Input: part model. Units: mm. Frame: model coordinates. Face numbers are marked on the shaded views. A direction names the side the tool comes from. Round coordinates to 2 decimals unless told otherwise and drop trailing zeros. Order: outer loops, then holes, each group sorted by start corner. A loop starts at its lowest first (then second) coordinate and runs counter-clockwise, first axis right, second up. Notation, with made-up numbers: (-38.5, 31.25) -> (-4.5, 31.25) arc R12 ccw to (-4.5, 41.25) -> close; hole circle Ø11 at (-5, -40). An arc over 180 degrees is marked (long way). Use a Markdown table: item, result.
from build123d import *

# Parameters (mm, degrees)
BOSS_EXTRUDE1_DEPTH = 6
FILLET1_R           = 20
SKETCH4_W           = 3
SKETCH4_H           = 8
SKETCH6_R           = 16.245672788
CUT_EXTRUDE1_DEPTH  = 10


with BuildPart() as part:
    # Sketch1 → Boss-Extrude1 (new body)
    with BuildSketch(Plane(origin=(0, 0, 0), x_dir=(1, 0, 0), z_dir=(0, 1, 0))):
        with BuildLine():
            Line((34.540516942, 38.609131748), (-36.459483058, 38.609131748))
            ThreePointArc((-36.459483058, 38.609131748), (-66.459483058, 1.109131748), (-36.459483058, -36.390868252))
            Line((-36.459483058, -36.390868252), (34.540516942, -36.390868252))
            ThreePointArc((34.540516942, -36.390868252), (64.540516942, 1.109131748), (34.540516942, 38.609131748))
        make_face()
    extrude(amount=BOSS_EXTRUDE1_DEPTH)

    # Fillet1
    fillet1_edges = [part.edges().sort_by_distance(p)[0] for p in [
        (-36.459483058, 3, -38.609131748),
        (34.540516942, 3, -38.609131748),
        (34.540516942, 3, 36.390868252),
        (-36.459483058, 3, 36.390868252),
    ]]
    fillet(fillet1_edges, radius=FILLET1_R)

    # Sweep1: sweep along a path in Sketch3
    with BuildLine(Plane.XZ) as sweep1_path:
        Line((31.907446823, 29.390868252), (-33.82641294, 29.390868252))
        ThreePointArc((-33.82641294, 29.390868252), (-35.899239553, 29.224550102), (-37.919027907, 28.729851303))
        ThreePointArc((-37.919027907, 28.729851303), (-59.459483058, -1.109131748), (-37.919027907, -30.948114799))
        ThreePointArc((-37.919027907, -30.948114799), (-35.899239553, -31.442813598), (-33.82641294, -31.609131748))
        Line((-33.82641294, -31.609131748), (31.907446823, -31.609131748))
        ThreePointArc((31.907446823, -31.609131748), (33.980273437, -31.442813598), (36.000061791, -30.948114799))
        ThreePointArc((36.000061791, -30.948114799), (57.540516942, -1.109131748), (36.000061791, 28.729851303))
        ThreePointArc((36.000061791, 28.729851303), (33.980273437, 29.224550102), (31.907446823, 29.390868252))
    # Sketch4 → Sweep1 (sweep)
    with BuildSketch(Plane(origin=(31.907446823, 0, -31.609131748), x_dir=(0, 0, -1), z_dir=(1, 0, 0))):
        with Locations((-1.5, -4)):
            Rectangle(SKETCH4_W, SKETCH4_H)
    sweep(path=sweep1_path.line)

    # Sketch6 → Cut-Extrude1 (cut)
    with BuildSketch(Plane(origin=(0, 0, 0), x_dir=(1, 0, 0), z_dir=(0, 1, 0))):
        with Locations((75, 0)):
            Circle(SKETCH6_R)
        with Locations((-76.918966117, 0)):
            Circle(SKETCH6_R)
    extrude(amount=CUT_EXTRUDE1_DEPTH, mode=Mode.SUBTRACT)


solid = part.part
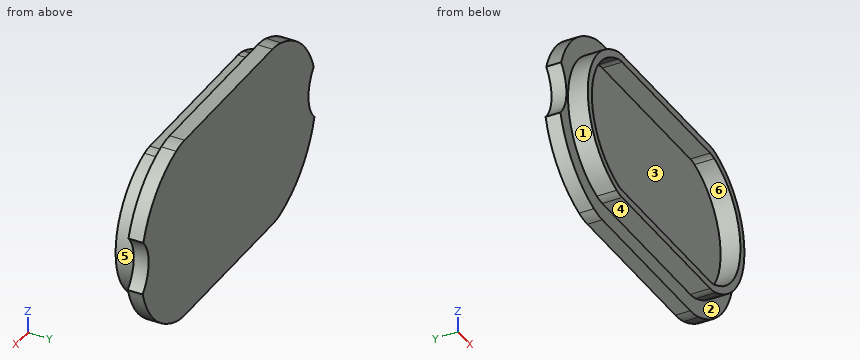
1) Cut plane B-B on x = -26. Return loops of the section in (y, z).
Results found:
| item | result |
|---|---|
| outline | (-8, -31.61) -> (0, -31.61) -> (0, -38.61) -> (6, -38.61) -> (6, 36.39) -> (0, 36.39) -> (0, 29.39) -> (-8, 29.39) -> (-8, 26.39) -> (0, 26.39) -> (0, -28.61) -> (-8, -28.61) -> close |
2) Cut plane C-C on z = -23.5. Return loops of the section in (x, y).
Results found:
| item | result |
|---|---|
| outline | (-59.26, 0) -> (-50.09, 0) -> (-50.09, -8) -> (-45.55, -8) -> (-45.55, 0) -> (43.63, 0) -> (43.63, -8) -> (48.17, -8) -> (48.17, 0) -> (57.35, 0) -> (57.35, 6) -> (-59.26, 6) -> close |
3) Cut plane A-A on y = -6.75. Return loops of the section in (x, z) (1 decimal).
Results found:
| item | result |
|---|---|
| outline | (-37.9, -30.9) arc R13 ccw to (-33.8, -31.6) -> (31.9, -31.6) arc R13 ccw to (36, -30.9) arc R31.4 ccw to (36, 28.7) arc R13 ccw to (31.9, 29.4) -> (-33.8, 29.4) arc R13 ccw to (-37.9, 28.7) arc R31.4 ccw to start; hole (-37, -28.1) arc R10 ccw to (-33.8, -28.6) -> (31.9, -28.6) arc R10 ccw to (35.1, -28.1) arc R28.4 ccw to (35.1, 25.9) arc R10 ccw to (31.9, 26.4) -> (-33.8, 26.4) arc R10 ccw to (-37, 25.9) arc R28.4 ccw to start |
4) Pin query (flat end, axial travel): pin 1 Ø4 at (x, y) = (13, -4.5) entering from +Z; pin 2 Ø2.5 at (x, y) = (-16.5, -4.5) entering from -Z; pin 3 Ø3 at (x, y) = (-46.5, 0) entering from -Z. Return the tip coordinate at first contact, or that it passes through.
Results found:
| item | result |
|---|---|
| pin 1 | stops at z = 29.39 |
| pin 2 | stops at z = -31.61 |
| pin 3 | stops at z = -35.59 |
5) Line query: L1, parallel to Z at x = 30.5, y = -2.5; L2, parallel to Y at x = -37, z = 17; L3, parallel to Z at x = -52, y = -1. Output: solid intervals per line, ascending. Write a range as [from, to].
Results found:
| item | result |
|---|---|
| L1 | z = [-31.61, -28.61], [26.39, 29.39] |
| L2 | y = [0, 6] |
| L3 | z = [-21.44, -16.4], [14.18, 19.22] |
6) Pull-direction query (X, two-part tool) for the marked faces 1, 2 and 3; classes: +X half, -X half, draft (parallel to the pull), parting line (faces both ways), or undercut.
Results found:
| item | result |
|---|---|
| face 1 | -X half |
| face 2 | draft |
| face 3 | undercut |
7) Set-up query: the marked faces 4, 5 and 6. Return all of +Z, -Z, +X, -X, +Y, -Y with unobstructed straight access to the full face (end or side cutting, diameter ignored); none if empty.
Results found:
| item | result |
|---|---|
| face 4 | -Z, +X, -X, -Y |
| face 5 | +X, -Y |
| face 6 | -Y |
